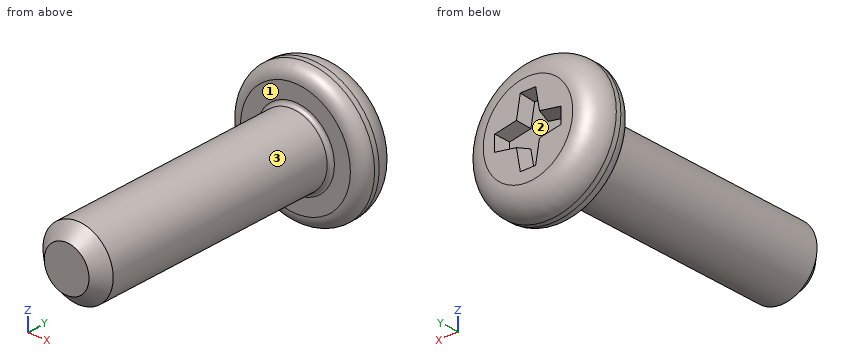
```python
from build123d import *

# Parameters (mm, degrees)
CUT_EXTRUDE1_DEPTH = 0.5
CUT_EXTRUDE1_TAPER = 15


with BuildPart() as part:
    # Sketch1 → Revolve1 (revolve)
    with BuildSketch(Plane.XY):
        with BuildLine():
            Line((0, -11.6), (0.875, -11.6))
            Line((0.875, -11.6), (1.375, -11.1))
            Line((1.375, -11.1), (1.375, -1.75))
            ThreePointArc((1.375, -1.75), (1.418933983, -1.643933983), (1.525, -1.6))
            Line((1.525, -1.6), (2.15, -1.6))
            ThreePointArc((2.15, -1.6), (2.503553391, -1.453553391), (2.65, -1.1))
            Line((2.65, -1.1), (2.65, -0.9))
            ThreePointArc((2.65, -0.9), (2.386396103, -0.263603897), (1.75, 0))
            Line((1.75, 0), (0, 0))
            Line((0, 0), (0, -11.6))
        make_face()
    revolve(axis=Axis((0, 0, 0), (0, -1, 0)))

    # Sketch2 → Cut-Extrude1 (cut)
    with BuildSketch(Plane(origin=(0, 0, 0), x_dir=(1, 0, 0), z_dir=(0, 1, 0))):
        Polygon((-0.300122066, 1.3), (-0.45, 0.45), (-1.3, 0.300122066), (-1.3, -0.300122066), (-0.45, -0.45), (-0.300122066, -1.3), (0.300122066, -1.3), (0.45, -0.45), (1.3, -0.300122066), (1.3, 0.300122066), (0.45, 0.45), (0.300122066, 1.3), align=None)
    extrude(amount=-CUT_EXTRUDE1_DEPTH, taper=CUT_EXTRUDE1_TAPER, mode=Mode.SUBTRACT)


solid = part.part
```
Design review of the part built by this model. Coordinates are the model's own, in mm. Face numbers are marked on the shaded views. Give positions to 0.01 mm unless a question says otherwise; leave off trailing zeros. Loops run counter-clockwise (first coordinate to the right, second up) from the corner with the lowest first, then second, coordinate; pieces in that order, holes last. Notation, with made-up numbers: M 44,67.25 L 103,67.25 A9 cw 103,82.25 Z; hole C 30.25,64 d8. An arc over 180 degrees is marked long. Return JSON: item names as keys, results as strings. Group by question number.
Item 1: We need section A-A (y = -2.75). Give the boundary of the cut face in (x, z) (3 decimals).
Item 2: Mouldability with a two-part tool opening along X and no side actions: class the marked faces 1, 2 and 3 as released by +X, released by -X, zero draft, split by the parting line, or undercut.
Item 3: For probe 1 along Y at (x, z) = (-0.35, 0); probe 2 along Z at (x, y) = (-0.9, -0.25); probe 3 along X at (y, z) = (-2.75, -0.45), list the stretches that pass through material, from the lowest coordinate up.
Item 4: We need section B-B (y = -1.25). Give the boundary of the cut face in (x, z).
Item 5: Insertion check: pin 1 Ø2 at (y, z) = (-4.5, 1.5) entering from -X; pin 2 Ø3 at (y, z) = (-5.5, -1) entering from +X (3 decimals); pin 3 Ø1.5 at (y, z) = (-3, -1) entering from -X. Each pin has a flat end and moves straight along its axis. Give the tip position at first contact, or say it passes through.
Output:
{
 "1": {"outline": "C 0,0 d2.75"},
 "2": {"face 1": "zero draft", "face 2": "undercut", "face 3": "split by the parting line"},
 "3": {"probe 1": "y = -11.6 to -0.5", "probe 2": "z = -2.2 to -0.3, 0.3 to 2.2", "probe 3": "x = -1.3 to 1.3"},
 "4": {"outline": "C 0,0 d5.25"},
 "5": {"pin 1": "stops at x = -1.28", "pin 2": "stops at x = 1.375", "pin 3": "stops at x = -1.35"}
}
